Source: CAD feature listing. Evaluate the final solid. Frame: model axes, mm. A direction names the side the tool comes from. Round coordinates to 2 decimals unless told otherwise and drop trailing zeros. Loops run counter-clockwise (first coordinate to the right, second up) from the corner with the lowest first, then second, coordinate; pieces in that order, holes last. Notation, with made-up numbers: (-25, 74.25) -> (9, 74.25) arc R28 ccw to (9, 112.25) -> close; hole circle Ø4 at (37, 68.25). An arc over 180 degrees is marked (long way). Return JSON: item names as keys, results as strings. Group by question number.
```python
from build123d import *
from build123d.topology import SkipClean

# Parameters (mm, degrees)
BOSS_EXTRUDE1_DEPTH               = 101.6
SKETCH3_R                         = 5.87375
CUT_EXTRUDE1_DEPTH                = 168.856337682
BOSS_EXTRUDE3_DEPTH               = 3.175
CUT_EXTRUDE2_DEPTH                = 3.96875
SKETCH5_R                         = 3.2385
CUT_EXTRUDE3_DEPTH                = 171.445522471
BOSS_EXTRUDE4_START               = -3.175
SKETCH7_R                         = 26.8097
SKETCH7_R_2                       = 5.87375
BOSS_EXTRUDE4_DEPTH               = 3.175
SKETCH6_R                         = 1.7272
CUT_EXTRUDE4_DEPTH                = 175.91949374
SKETCH8_W                         = 12.7
SKETCH8_H                         = 12.7
SKETCH8_R                         = 3.2385
BOSS_EXTRUDE5_DEPTH               = 12.7
CUT_EXTRUDE5_DEPTH                = 175.91949374
CUT_EXTRUDE5_DEPTH_BACK           = 175.91949374
SKETCH10_R                        = 15.8369
SKETCH13_W                        = 4.8895
SKETCH13_H                        = 11.125454
CUT_EXTRUDE7_DEPTH                = 9.8425
F_10_0_1935_DIAMETER_HOLE1_REACH  = 160.559
F_10_0_1935_DIAMETER_HOLE1_BORE_R = 2.48285


with BuildPart() as part:
    # Sketch2 → Boss-Extrude1 (new body)
    with BuildSketch(Plane.XY):
        Polygon((0, 78.74), (0, 0), (107.95, 0), (107.95, 78.74), (104.775, 78.74), (104.775, 12.7), (3.175, 12.7), (3.175, 78.74), align=None)
    extrude(amount=BOSS_EXTRUDE1_DEPTH)

    # Sketch3 → Cut-Extrude1 (cut, through all)
    with BuildSketch(Plane.ZY):
        with BuildLine():
            ThreePointArc((0, 19.05), (0.495062251, 23.364717272), (1.954518124, 27.455176943))
            Line((1.954518124, 27.455176943), (26.740958507, 77.868885684))
            ThreePointArc((26.740958507, 77.868885684), (26.961098465, 78.306490439), (27.189197089, 78.74))
            Line((27.189197089, 78.74), (0, 78.74))
            Line((0, 78.74), (0, 19.05))
        make_face()
        with BuildLine():
            Line((101.6, 78.74), (74.410802911, 78.74))
            ThreePointArc((74.410802911, 78.74), (74.638901535, 78.306490439), (74.859041493, 77.868885684))
            Line((74.859041493, 77.868885684), (99.645481876, 27.455176943))
            ThreePointArc((99.645481876, 27.455176943), (101.104937749, 23.364717272), (101.6, 19.05))
            Line((101.6, 19.05), (101.6, 78.74))
        make_face()
        with Locations(Location((50.8, 66.04, 0), (0, 0, 270))):
            Circle(SKETCH3_R)
    extrude(amount=-CUT_EXTRUDE1_DEPTH, mode=Mode.SUBTRACT)

    # Sketch3_4 → Boss-Extrude3 (add)
    with SkipClean():  # the faces are left unmerged after this step: merging them gives an invalid solid
        with BuildSketch(Plane.ZY):
            with BuildLine():
                ThreePointArc((74.410802911, 78.74), (50.8, 92.8497), (27.189197089, 78.74))
                Line((27.189197089, 78.74), (74.410802911, 78.74))
            make_face()
        extrude(amount=-BOSS_EXTRUDE3_DEPTH)

    # Sketch4 → Cut-Extrude2 (cut)
    with SkipClean():  # the faces are left unmerged after this step: merging them gives an invalid solid
        with BuildSketch(Plane(origin=(0, 12.7, 0), x_dir=(1, 0, 0), z_dir=(0, 1, 0))):
            Polygon((60.325, -47.133825791), (53.975, -43.467651581), (47.625, -47.133825791), (47.625, -54.466174209), (53.975, -58.132348419), (60.325, -54.466174209), align=None)
        extrude(amount=-CUT_EXTRUDE2_DEPTH, mode=Mode.SUBTRACT)

    # Sketch5 → Cut-Extrude3 (cut, through all)
    with SkipClean():  # the faces are left unmerged after this step: merging them gives an invalid solid
        with BuildSketch(Plane(origin=(0, 8.73125, 0), x_dir=(1, 0, 0), z_dir=(0, 1, 0))):
            with Locations(Location((53.975, -50.8, 0), (0, 0, 180))):
                Circle(SKETCH5_R)
        extrude(amount=-CUT_EXTRUDE3_DEPTH, mode=Mode.SUBTRACT)

    # Sketch7 → Boss-Extrude4 (add)
    with SkipClean():  # the faces are left unmerged after this step: merging them gives an invalid solid
        with BuildSketch(Plane(origin=(107.95, 0, 0), x_dir=(0, 0, -1), z_dir=(1, 0, 0)).offset(BOSS_EXTRUDE4_START)):
            with Locations((-50.8, 66.04)):
                Circle(SKETCH7_R)
            with Locations(Location((-50.8, 66.04, 0), (0, 0, 270))):
                Circle(SKETCH7_R_2, mode=Mode.SUBTRACT)
        extrude(amount=BOSS_EXTRUDE4_DEPTH)

    # Sketch6 → Cut-Extrude4 (cut, through all)
    with SkipClean():  # the faces are left unmerged after this step: merging them gives an invalid solid
        with BuildSketch(Plane.ZY):
            with Locations(Location((32.65297, 76.5175, 0), (0, 0, 270))):
                Circle(SKETCH6_R)
            with Locations(Location((68.94703, 76.5175, 0), (0, 0, 270))):
                Circle(SKETCH6_R)
            with Locations(Location((50.8, 30.480783465, 0), (0, 0, 270))):
                Circle(SKETCH6_R)
        extrude(amount=-CUT_EXTRUDE4_DEPTH, mode=Mode.SUBTRACT)

    # Sketch8 → Boss-Extrude5 (add)
    with SkipClean():  # the faces are left unmerged after this step: merging them gives an invalid solid
        with BuildSketch(Plane.XZ):
            with Locations((53.975, 50.8)):
                Rectangle(SKETCH8_W, SKETCH8_H)
            with Locations(Location((53.975, 50.8, 0), (0, 0, 180))):
                Circle(SKETCH8_R, mode=Mode.SUBTRACT)
        extrude(amount=BOSS_EXTRUDE5_DEPTH)

    # Sketch9 → Revolve1 (revolve)
    with SkipClean():  # the faces are left unmerged after this step: merging them gives an invalid solid
        with BuildSketch(Plane.ZY.offset(-53.975), mode=Mode.PRIVATE) as revolve1_sk:
            Polygon((44.45, -12.7), (44.45, 0), (31.75, 0), (41.3385, -12.7), align=None)
        revolve(revolve1_sk.sketch.rotate(Axis((53.975, -12.7, 50.8), (0, 1, 0)), 90), axis=Axis((53.975, -12.7, 50.8), (0, 1, 0)))

    # Sketch10 → Cut-Extrude5 (cut, two sides: drawn at the far end of the back side and taken through both)
    with SkipClean():  # the faces are left unmerged after this step: merging them gives an invalid solid
        with BuildSketch(Plane(origin=(107.95, 0, 0), x_dir=(0, 0, -1), z_dir=(1, 0, 0)).offset(-CUT_EXTRUDE5_DEPTH_BACK)):
            with Locations(Location((-50.8, 66.04, 0), (0, 0, 90))):
                Circle(SKETCH10_R)
        extrude(amount=CUT_EXTRUDE5_DEPTH + CUT_EXTRUDE5_DEPTH_BACK, mode=Mode.SUBTRACT)

    # Sketch13 → Cut-Extrude7 (cut)
    with SkipClean():  # the faces are left unmerged after this step: merging them gives an invalid solid
        with BuildSketch(Plane.XZ):
            with Locations((90.83675, 76.2)):
                Rectangle(SKETCH13_W, SKETCH13_H)
            with Locations((90.83675, 25.4)):
                Rectangle(SKETCH13_W, SKETCH13_H)
        cut_extrude7 = extrude(amount=-CUT_EXTRUDE7_DEPTH, mode=Mode.SUBTRACT)

    # 10 _0.1935_ Diameter Hole1 bore (on position points) → 10 _0.1935_ Diameter Hole1 (cut, up to next)
    with BuildSketch(Plane(origin=(107.95, 5.207, 76.2), x_dir=(0, 1, 0), z_dir=(1, 0, 0)), mode=Mode.PRIVATE) as f_10_0_1935_diameter_hole1_sk1:
        Circle(F_10_0_1935_DIAMETER_HOLE1_BORE_R)
    f_10_0_1935_diameter_hole1_tool1 = extrude(f_10_0_1935_diameter_hole1_sk1.sketch, amount=-F_10_0_1935_DIAMETER_HOLE1_REACH, mode=Mode.PRIVATE) & part.part
    # 10 _0.1935_ Diameter Hole1 bore (on position points) → 10 _0.1935_ Diameter Hole1 (cut, up to next)
    with BuildSketch(Plane(origin=(107.95, 5.207, 76.2), x_dir=(0, 1, 0), z_dir=(1, 0, 0)), mode=Mode.PRIVATE) as f_10_0_1935_diameter_hole1_sk2:
        with Locations((0, -50.8)):
            Circle(F_10_0_1935_DIAMETER_HOLE1_BORE_R)
    f_10_0_1935_diameter_hole1_tool2 = extrude(f_10_0_1935_diameter_hole1_sk2.sketch, amount=-F_10_0_1935_DIAMETER_HOLE1_REACH, mode=Mode.PRIVATE) & part.part
    f_10_0_1935_diameter_hole1_1 = f_10_0_1935_diameter_hole1_tool1.solids().sort_by_distance((107.95, 5.207, 76.2))[0]
    add(f_10_0_1935_diameter_hole1_1, mode=Mode.SUBTRACT)
    f_10_0_1935_diameter_hole1_2 = f_10_0_1935_diameter_hole1_tool2.solids().sort_by_distance((107.95, 5.207, 25.4))[0]
    add(f_10_0_1935_diameter_hole1_2, mode=Mode.SUBTRACT)
    f_10_0_1935_diameter_hole1 = f_10_0_1935_diameter_hole1_1 + f_10_0_1935_diameter_hole1_2  # 10 _0.1935_ Diameter Hole1 as one shape, for the pattern or mirror that repeats it

    # Mirror2: Cut-Extrude7, 10 _0.1935_ Diameter Hole1 across plane
    with SkipClean():  # the faces are left unmerged after this step: merging them gives an invalid solid
        add(cut_extrude7.mirror(Plane(origin=(53.975, 0, 0), x_dir=(0, 0, 1), z_dir=(1, 0, 0))), mode=Mode.SUBTRACT)
        add(f_10_0_1935_diameter_hole1.mirror(Plane(origin=(53.975, 0, 0), x_dir=(0, 0, 1), z_dir=(1, 0, 0))), mode=Mode.SUBTRACT)


solid = part.part
```
(1) Cut plane D-D (z = 50.8). Count the separate pieces of the cut face and the enclosed holes in it, and give its area (3 significant figures).
(2) Cut plane C-C (y = 66.04). Return loops of the section in (x, z) (3 decimals).
(3) Pin query (flat end, axial travel): pin 1 (5 mm diameter, centred on x = 79, z = 58, fed in from -Y); pin 2 (1.5 mm diameter, centred on x = 80.5, y = 15, fed in from -Z); pin 3 (6 mm diameter, centred on x = 60.5, z = 80.5, fed in from +Y); pin 4 (4 mm diameter, centred on y = 5.207, z = 25.4, fed in from +X). Return the tip coordinate at first contact, or that it passes through.
(4) Cut plane A-A (x = 96.5). Return loops of the section in (y, z), and give its area (3 significant figures).
(5) Set-up query: faces 1 (the face through (7.232, 3.237, 23.889)), 2 (the face through (14.669, 2.7, 74.9)), 3 (the face through (43, 12.7, 50)), 4 (the face through (100.718, 4.669, 73.776)), 5 (the face through (50.8, 10.7, 56.3)). Return all of +Z, -Z, +X, -X, +Y, -Y with unobstructed straight access to the full face (end or side cutting, diameter ignored); none if empty.
(6) Cut plane B-B (y = 16). Return loops of the section in (x, z) (3 decimals).
(7) Ray query, line 1 (X direction, y = 77, z = 65.5) (3 decimals); line 2 (Y direction, x = 9, z = 9); line 3 (Z direction, x = 106, y = 66). Return the intervals inside material, ascending.
(8) Mould query, pull axis Z, two halves, no side actions, for faces 6 (the face through (17, 5, 19.837)), 7 (the face through (0, 37, 50)), 8 (the face through (53, 8, 101.6)). Classes: released by +Z, released by -Z, zero draft, split by the parting line, or undercut.
Answers follow:
{
 "1": {"separate pieces": "6", "enclosed holes": "0", "area": "1,830 mm^2"},
 "2": {"outline": "(0, 20.925) -> (3.175, 20.925) -> (3.175, 34.963) -> (0, 34.963) -> close; (0, 66.637) -> (3.175, 66.637) -> (3.175, 80.675) -> (0, 80.675) -> close; (104.775, 20.925) -> (107.95, 20.925) -> (107.95, 34.963) -> (104.775, 34.963) -> close; (104.775, 66.637) -> (107.95, 66.637) -> (107.95, 80.675) -> (104.775, 80.675) -> close"},
 "3": {"pin 1": "y = 0", "pin 2": "through", "pin 3": "y = 12.7", "pin 4": "x = 88.39"},
 "4": {"outline": "(0, 0) -> (12.7, 0) -> (12.7, 101.6) -> (0, 101.6) -> close; hole circle Ø4.97 at (5.21, 25.4); hole circle Ø4.97 at (5.21, 76.2)", "area": "1,250 mm^2"},
 "5": {"face 1": "-X", "face 2": "-Y", "face 3": "+Z, -Z, +Y", "face 4": "+X", "face 5": "+Y"},
 "6": {"outline": "(0, 0) -> (3.175, 0) -> (3.175, 101.6) -> (0, 101.6) -> close; (104.775, 0) -> (107.95, 0) -> (107.95, 101.6) -> (104.775, 101.6) -> close"},
 "7": {"line 1": "0 to 3.175, 104.775 to 107.95", "line 2": "0 to 12.7", "line 3": "20.91 to 34.96, 66.64 to 80.69"},
 "8": {"face 6": "undercut", "face 7": "zero draft", "face 8": "released by +Z"}
}
